For this review, take the finished solid that the model builds, in its own axes (mm). A direction names the side the tool comes from. Round coordinates to 2 decimals unless told otherwise and drop trailing zeros. Order: outer loops, then holes, each group sorted by start corner. A loop starts at its lowest first (then second) coordinate and runs counter-clockwise, first axis right, second up. Notation, with made-up numbers: (88, -2.5) - (108, -2.5) arc R20 ccw to (108, 25.5) - close; hole circle Ø1 at (51.5, 4). An arc over 180 degrees is marked (long way). One line per item, written item: value.
Autodesk Fusion 360 part; units mm, degrees
sketch "Sketch2" plane through (0, 0, 0) normal (0, 0, 1) x (1, 0, 0)
  line L0 (8, -13) -> (-8, -13)
  line L1 (-8, -13) -> (-8, 13)
  line L2 (-8, 13) -> (8, 13)
  line L3 (8, 13) -> (8, -13)
  line L4 (8, -13) -> (-8, 13) construction
  line L5 (-8, -13) -> (8, 13) construction
  line L6 (3, -5.5) -> (-3, -5.5)
  line L7 (-3, -5.5) -> (-3, 5.5)
  line L8 (-3, 5.5) -> (3, 5.5)
  line L9 (3, 5.5) -> (3, -5.5)
  line L10 (3, -5.5) -> (-3, 5.5) construction
  line L11 (-3, -5.5) -> (3, 5.5) construction
  dimension "d23" = 16
  dimension "d24" = 26
  dimension "d25" = 6
  dimension "d26" = 11
extrude "Extrude2" add sketch "Sketch2" along normal blind 3
fillet "Fillet6" radius 2 4 edges at (8, 13, 1.5) (-8, 13, 1.5) (-8, -13, 1.5) (8, -13, 1.5)
fillet "Fillet7" radius 2.25 4 edges at (-3, 5.5, 1.5) (3, 5.5, 1.5) (3, -5.5, 1.5) (-3, -5.5, 1.5)
extrude "Extrude1" [suppressed]
fillet "Fillet1" [suppressed]
fillet "Fillet2" [suppressed]
fillet "Fillet3" [suppressed]
fillet "Fillet4" [suppressed]
fillet "Fillet5" [suppressed]
Item 1: Wall thickness on line 1 (Y direction, x = 0, z = 1.6); line 2 (X direction, y = 2.25, z = 0.5); line 3 (Y direction, x = -2, z = 1.7): over which ranges is each line inside the solid? List them lowest first.
Returned:
line 1: -13 to -5.5, 5.5 to 13
line 2: -8 to -3, 3 to 8
line 3: -13 to -5.12, 5.12 to 13
Item 2: Take a section at B-B (z = 0.35). Write out the cut boundary in (x, y), plus the area to 3 significant figures.
Returned:
outline: (-8, -11) arc R2 ccw to (-6, -13) - (6, -13) arc R2 ccw to (8, -11) - (8, 11) arc R2 ccw to (6, 13) - (-6, 13) arc R2 ccw to (-8, 11) - close; hole (-3, -3.25) arc R2.25 ccw to (-0.75, -5.5) - (0.75, -5.5) arc R2.25 ccw to (3, -3.25) - (3, 3.25) arc R2.25 ccw to (0.75, 5.5) - (-0.75, 5.5) arc R2.25 ccw to (-3, 3.25) - close
area: 351 mm^2
Item 3: The part is to be moulded in two halves that separate along Y. For faces 3 (the flat face through (0, 5.5, 1)), 4 (the flat face through (-8, 0, 1)), 5 (the cylindrical face through (-7.43, -12.4, 1.52)), say which applies: +Y half, -Y half, draft (parallel to the pull), parting line (faces both ways), or undercut.
Returned:
face 3: undercut
face 4: draft
face 5: -Y half
Item 4: Machinability: for faces 1 (the cylindrical face through (7.43, 12.4, 1.52)), 2 (the flat face through (-3, 0, 1)), which of the approach directions +Z, -Z, +X, -X, +Y, -Y give a long, thin tool a straight path to every point of the face, cutting with its end or side? Answer none if there is none.
Returned:
face 1: +Z, -Z, +X, +Y
face 2: +Z, -Z
Item 5: Take a section at D-D (x = 7). Write out the cut boundary in (y, z), plus the area to 3 significant figures.
Returned:
outline: (-12.73, 0) - (12.73, 0) - (12.73, 3) - (-12.73, 3) - close
area: 76.4 mm^2
Item 6: Take a section at C-C (x = -0.25). Write out the cut boundary in (y, z), plus the area to 3 significant figures.
Returned:
outline: (-13, 0) - (-5.5, 0) - (-5.5, 3) - (-13, 3) - close; (5.5, 0) - (13, 0) - (13, 3) - (5.5, 3) - close
area: 45.0 mm^2
Item 7: Take a section at A-A (y = -0.5). Write out the cut boundary in (x, z), plus the area to 3 significant figures.
Returned:
outline: (-8, 0) - (-3, 0) - (-3, 3) - (-8, 3) - close; (3, 0) - (8, 0) - (8, 3) - (3, 3) - close
area: 30.0 mm^2
Item 8: For P1, Ø5, axis at x = 1, y = -10.5, coming from the -Z side, flat-tipped, find the tip position at first contact; note if it passes through.
Returned:
P1: z = 0
